Work out the finished part from the listing and answer in its coordinate system (mm). A direction names the side the tool comes from. Round coordinates to 2 decimals unless told otherwise and drop trailing zeros. Write each loop counter-clockwise with the first axis right and the second up, starting at its lowest first coordinate (ties: lowest second). Pieces come first, ordered by that corner, then holes.
from build123d import *

# Parameters (mm, degrees)
SKETCH1_R           = 3.175
BOSS_EXTRUDE1_DEPTH = 5.461
SKETCH3_W           = 4.7625
SKETCH3_H           = 33.783
SKETCH3_H_2         = 46.289475607
CUT_EXTRUDE2_DEPTH  = 10


with BuildPart() as part:
    # Sketch1 → Boss-Extrude1 (new body)
    with BuildSketch(Plane(origin=(0, 0, 0), x_dir=(1, 0, 0), z_dir=(0, 1, 0))):
        with BuildLine():
            Line((0, 0), (-83.629476528, 83.629476528))
            ThreePointArc((-83.629476528, 83.629476528), (-85.081850373, 100.91197572), (-70.310188895, 110))
            Line((-70.310188895, 110), (-56.601944845, 110))
            Line((-56.601944845, 110), (0, 94.833554589))
            Line((0, 94.833554589), (0, 58.293))
            Line((0, 58.293), (8, 58.293))
            Line((8, 58.293), (8, -58.293))
            Line((8, -58.293), (0, -58.293))
            Line((0, -58.293), (0, -94.833554589))
            Line((0, -94.833554589), (-56.601944845, -110))
            Line((-56.601944845, -110), (-70.310188895, -110))
            ThreePointArc((-70.310188895, -110), (-85.081850373, -100.91197572), (-83.629476528, -83.629476528))
            Line((-83.629476528, -83.629476528), (0, 0))
        make_face()
        with Locations((-70.310188895, 93.451069294)):
            Circle(SKETCH1_R, mode=Mode.SUBTRACT)
        with Locations((-70.310188895, -93.451069294)):
            Circle(SKETCH1_R, mode=Mode.SUBTRACT)
    extrude(amount=BOSS_EXTRUDE1_DEPTH)

    # Sketch3 → Cut-Extrude2 (cut)
    with BuildSketch(Plane(origin=(0, 0, 0), x_dir=(1, 0, 0), z_dir=(0, 1, 0))):
        Polygon((-4.829629131, 96.127649814), (-17.19282542, 99.440358276), (-18.425451123, 94.840136528), (-6.062254834, 91.527428067), align=None)
        Polygon((-24.920232031, 101.510910637), (-37.283428319, 104.823619098), (-38.516054022, 100.22339735), (-26.152857733, 96.910688889), align=None)
        with Locations((5.61875, 33.4015)):
            Rectangle(SKETCH3_W, SKETCH3_H)
        Polygon((-26.152857733, -96.910688889), (-38.516054022, -100.22339735), (-37.283428319, -104.823619098), (-24.920232031, -101.510910637), align=None)
        Polygon((-6.062254834, -91.527428067), (-18.425451123, -94.840136528), (-17.19282542, -99.440358276), (-4.829629131, -96.127649814), align=None)
        with Locations((5.61875, -39.654737804)):
            Rectangle(SKETCH3_W, SKETCH3_H_2)
    extrude(amount=CUT_EXTRUDE2_DEPTH, mode=Mode.SUBTRACT)


solid = part.part
Q1. Given pin 1 (2.5 mm diameter, centred on x = 6.5, y = 3, fed in from -Z); pin 2 (5.5 mm diameter, centred on x = -70.31, z = -93.45, fed in from -Y); pin 3 (2.5 mm diameter, centred on y = 4, z = 73, fed in from +X); pin 4 (3 mm diameter, centred on y = 4.5, z = 67.5, fed in from -X), each flat-ended and moving along its own axis, determine where each tip first touches the part or whether it passes through.
Q2. A tool of negligible diameter and unlimited length cuts with its end or side. For faces 1 (the face through (-25.545, 2.692, -99.179)), 2 (the face through (8, 3, -54)), 3 (the face through (4, 3, -58.293)), 4 (the face through (6, 3, -50.293)), 5 (the face through (3.238, 3, 38)), from which of +Z, -Z, +X, -X, +Y, -Y can it reach the whole face along a straight path? Write none if from no direction.
Q3. The mould has two halves that part along Z. Classify faces 6 (the face through (-68.85, 2.69, 96.27)), 7 (the face through (-5.455, 2.692, -93.795)), 8 (the face through (6, 3, 16.51)): +Z half, -Z half, draft (parallel to the pull), parting line (faces both ways), or undercut.
Q4. Find section C-C (x = -44.5). Determine the outline of the cut face in (y, z).
Q5. Find the intervals of material crossed by L1, parallel to Z at x = -4.5, y = 4.6; L2, parallel to Z at x = -52, y = 2.75; L3, parallel to X at y = 1.05, z = -85.5, in increasing order.
Q6. Find section A-A (x = -62). Determine the outline of the cut face in (y, z), plus the area to 3 significant figures.
Q7. Find section D-D (y = 1.1). Count the separate pieces of the cut face and the enclosed holes in it, plus the area to 3 significant figures.
Q8. Find section B-B (z = -39). Determine the outline of the cut face in (x, y).
Report:
1. pin 1: stops at z = -58.29
1. pin 2: passes through
1. pin 3: stops at x = 0
1. pin 4: stops at x = -69
2. face 1: -Z, +Y, -Y
2. face 2: +Z, -Z, +X, +Y, -Y
2. face 3: -Z, +X, +Y, -Y
2. face 4: +X, +Y, -Y
2. face 5: +Z, +X, +Y, -Y
3. face 6: undercut
3. face 7: -Z half
3. face 8: +Z half
4. outline: (0, -106.76) - (5.46, -106.76) - (5.46, -44.5) - (0, -44.5) - close; (0, 44.5) - (5.46, 44.5) - (5.46, 106.76) - (0, 106.76) - close
5. L1: z = -96.04 to -4.5, 4.5 to 96.04
5. L2: z = -108.77 to -52, 52 to 108.77
5. L3: x = -84.82 to 0
6. outline: (0, -110) - (5.46, -110) - (5.46, -62) - (0, -62) - close; (0, 62) - (5.46, 62) - (5.46, 110) - (0, 110) - close
6. area: 524 mm2
7. separate pieces: 1
7. enclosed holes: 2
7. area: 10,800 mm2
8. outline: (-39, 0) - (3.24, 0) - (3.24, 5.46) - (-39, 5.46) - close
